Input: part model. Units: mm. Frame: model coordinates. A direction names the side the tool comes from. Give positions to 0.01 mm unless a question says otherwise; leave off trailing zeros. Loops run counter-clockwise (first coordinate to the right, second up) from the corner with the lowest first, then second, coordinate; pieces in that order, holes last. Notation, with made-up numbers: (-19.75, -36) -> (27.25, -36) arc R20 ccw to (27.25, -23) -> close; hole circle Ø8 at (51.25, 77.25). An arc over 180 degrees is marked (long way). One line per question, with ' | ' between items.
from build123d import *

# Parameters (mm, degrees)
F0_W          = 55.7
F0_H          = 13.4
F1_DEPTH      = 1.6
F2_W          = 55.7
F2_H          = 13.4
F2_W_2        = 26
F2_H_2        = 6
F3_DEPTH      = 4
F4_W          = 8
F4_H          = 10
F5_DEPTH      = 3
F6_T1_DEPTH   = 70.7
F7_W          = 6
F7_H          = 3.5
F8_DEPTH      = 10
F9_R          = 2
F10_T4_DEPTH  = 21.4300979278
F10_T10_DEPTH = 41.4300979278
F10_T16_DEPTH = 41.4300979278
F10_T22_DEPTH = 21.4300979278
F11_C1_SIZE   = 2
F11_C2_SIZE   = 2


# Not quite as in the source:
# - a fillet or chamfer that OpenCascade refuses, or shapes differently, is made with other operations: its cross-section is extruded or revolved along the edge and cut away or added


with BuildPart() as f1:
    # F0 (on Top) → F1 (new body)
    with BuildSketch(Plane.XY):
        with Locations((-20.85, 5.5)):
            Rectangle(F0_W, F0_H)
        Polygon((1, 0), (0, 0), (-47.5, 0), (-47.5, 11), (0, 11), (1, 11), align=None, mode=Mode.SUBTRACT)
    extrude(amount=F1_DEPTH)

    # F2 (on face) → F3 (join)
    with BuildSketch(Plane.XY.offset(1.6)):
        with Locations((-20.85, 5.5)):
            Rectangle(F2_W, F2_H)
        Polygon((-47.5, 0.5), (-47.5, 10.5), (-47.5, 11), (1, 11), (1, 0), (-47.5, 0), align=None, mode=Mode.SUBTRACT)
        Polygon((-47.5, 11), (-47.5, 10.5), (-31.5, 10.5), (-31.5, 0.5), (-47.5, 0.5), (-47.5, 0), (1, 0), (1, 11), align=None)
        with Locations((-13, 5.5)):
            Rectangle(F2_W_2, F2_H_2, mode=Mode.SUBTRACT)
    extrude(amount=F3_DEPTH)

    # F4 (on face) → F5 (join)
    with BuildSketch(Plane.XY.offset(5.6)):
        Polygon((-39.5, 12.2), (-48.7, 12.2), (-48.7, -1.2), (-39.5, -1.2), (-39.5, 0.5), (-47.5, 0.5), (-47.5, 10.5), (-39.5, 10.5), align=None)
        with Locations((-43.5, 5.5)):
            Rectangle(F4_W, F4_H)
    extrude(amount=-F5_DEPTH)

    # F6: fillet of radius 3 on 2 edges, made by hand

    # F6_s2 → F6_t1 (cut)
    with BuildSketch(Plane.YZ.offset(-56.2)):
        with BuildLine():
            ThreePointArc((12.2, 2.6), (11.3213203436, 4.7213203436), (9.2, 5.6))
            Line((9.2, 5.6), (12.2, 5.6))
            Line((12.2, 5.6), (12.2, 2.6))
        make_face()
        with BuildLine():
            ThreePointArc((1.8, 5.6), (-0.3213203436, 4.7213203436), (-1.2, 2.6))
            Line((-1.2, 2.6), (-1.2, 5.6))
            Line((-1.2, 5.6), (1.8, 5.6))
        make_face()
    extrude(amount=F6_T1_DEPTH, mode=Mode.SUBTRACT)

    # F7 (on face) → F8 (cut)
    with BuildSketch(Plane(origin=(-48.7, 0, 0), x_dir=(0, -1, 0), z_dir=(-1, 0, 0))):
        with Locations((-5.5, 1.75)):
            Rectangle(F7_W, F7_H)
    extrude(amount=-F8_DEPTH, mode=Mode.SUBTRACT)

    # F9
    f9_edges = [f1.edges().sort_by_distance(p)[0] for p in [
        (-44.1, 8.5, 3.5),
        (-44.1, 2.5, 3.5),
    ]]
    fillet(f9_edges, radius=F9_R)

    # F10: chamfer of 3 on 4 edges, made by hand


with BuildPart() as f10_tool2:
    # F10_s3 → F10_t4 (new body)
    with BuildSketch(Plane.XZ.offset(5.2150489639)):
        Polygon((-29, 5.6), (-26, 2.6), (-26, 5.6), align=None)
    extrude(amount=-F10_T4_DEPTH)

    split(bisect_by=Plane(origin=(0, 2.55, 2.55), x_dir=(1, 0, 0), z_dir=(0, 0.7071067812, 0.7071067812)), keep=Keep.TOP)

    split(bisect_by=Plane(origin=(0, 2.95, -2.95), x_dir=(1, 0, 0), z_dir=(0, -0.7071067812, 0.7071067812)), keep=Keep.TOP)


with BuildPart() as f1_1:
    add(f1.part)

    # F10_t1: cut F10_tool2
    add(f10_tool2.part, mode=Mode.SUBTRACT)


with BuildPart() as f10_tool8:
    # F10_s9 → F10_t10 (new body)
    with BuildSketch(Plane.YZ.offset(-33.7150489639)):
        Polygon((11.5, 5.6), (8.5, 2.6), (8.5, 5.6), align=None)
    extrude(amount=F10_T10_DEPTH)

    split(bisect_by=Plane(origin=(-11.7, 0, -11.7), x_dir=(0, 1, 0), z_dir=(0.7071067812, 0, 0.7071067812)), keep=Keep.TOP)

    split(bisect_by=Plane(origin=(-1.3, 0, 1.3), x_dir=(0, 1, 0), z_dir=(-0.7071067812, 0, 0.7071067812)), keep=Keep.TOP)


with BuildPart() as f1_2:
    add(f1_1.part)

    # F10_t7: cut F10_tool8
    add(f10_tool8.part, mode=Mode.SUBTRACT)


with BuildPart() as f10_tool14:
    # F10_s15 → F10_t16 (new body)
    with BuildSketch(Plane.YZ.offset(7.7150489639)):
        Polygon((-0.5, 5.6), (2.5, 2.6), (2.5, 5.6), align=None)
    extrude(amount=-F10_T16_DEPTH)

    split(bisect_by=Plane(origin=(-11.7, 0, -11.7), x_dir=(0, 1, 0), z_dir=(0.7071067812, 0, 0.7071067812)), keep=Keep.TOP)

    split(bisect_by=Plane(origin=(-1.3, 0, 1.3), x_dir=(0, 1, 0), z_dir=(-0.7071067812, 0, 0.7071067812)), keep=Keep.TOP)


with BuildPart() as f1_3:
    add(f1_2.part)

    # F10_t13: cut F10_tool14
    add(f10_tool14.part, mode=Mode.SUBTRACT)


with BuildPart() as f10_tool20:
    # F10_s21 → F10_t22 (new body)
    with BuildSketch(Plane.XZ.offset(-16.2150489639)):
        Polygon((3, 5.6), (0, 2.6), (0, 5.6), align=None)
    extrude(amount=F10_T22_DEPTH)

    split(bisect_by=Plane(origin=(0, 2.55, 2.55), x_dir=(1, 0, 0), z_dir=(0, 0.7071067812, 0.7071067812)), keep=Keep.TOP)

    split(bisect_by=Plane(origin=(0, 2.95, -2.95), x_dir=(1, 0, 0), z_dir=(0, -0.7071067812, 0.7071067812)), keep=Keep.TOP)


with BuildPart() as f1_4:
    add(f1_3.part)

    # F10_t19: cut F10_tool20
    add(f10_tool20.part, mode=Mode.SUBTRACT)

    # F11: chamfer of 2 on 3 edges, made by hand

    # F11_c1
    f11_c1_edges = [f1_4.edges().sort_by_distance(p)[0] for p in [
        (-31.5, 5.5, 1.6),
    ]]
    chamfer(f11_c1_edges, length=F11_C1_SIZE)

    # F11_c2
    f11_c2_edges = [f1_4.edges().sort_by_distance(p)[0] for p in [
        (-39.5, 9.3351646544, 2.6),
    ]]
    chamfer(f11_c2_edges, length=F11_C2_SIZE)


solid = f1_4.part
1. Section query C-C (x = -35). Output: boundary loops of the cut face in (y, z).
Determined:
outline: (-1.2, 0) -> (0, 0) -> (0, 1.6) -> (0.5, 1.6) -> (0.5, 5.3) arc R3 ccw to (-1.2, 2.6) -> close; (10.5, 1.6) -> (11, 1.6) -> (11, 0) -> (12.2, 0) -> (12.2, 2.6) arc R3 ccw to (10.5, 5.3) -> close
2. Section query D-D (z = 0.85). Output: boundary loops of the cut face in (x, y), then the cut area to 3 significant figures.
Determined:
outline: (-48.7, -1.2) -> (7, -1.2) -> (7, 12.2) -> (-48.7, 12.2) -> (-48.7, 8.5) -> (-47.5, 8.5) -> (-47.5, 11) -> (1, 11) -> (1, 0) -> (-47.5, 0) -> (-47.5, 2.5) -> (-48.7, 2.5) -> close | area: 206 mm2
3. Pin query (flat end, axial travel): P1, Ø0.5, axis at y = 5.5, z = 2, coming from the -X side; P2, Ø1.9, axis at x = -46, y = 9.5, coming from the -Z side; P3, Ø1.9, axis at x = -39.5, z = 3.5, coming from the +Y side; P4, Ø0.8, axis at y = 8, z = 0.5, coming from the -X side. Return the tip coordinate at first contact, or that it passes through.
Determined:
P1: stops at x = -30.15 | P2: stops at z = 2.6 | P3: stops at y = 12.2 | P4: stops at x = 1
4. Reachability of faces 1 (the flat face through (-18, 2, 1.6)), 2 (the cylindrical face through (-44.6, 3.3, 3.1)), 3 (the flat face through (0, 5, 2)) from +Z, -Z, +X, -X, +Y, -Y: full face, straight path, thin tool, end or side. Return the list, or none.
Determined:
face 1: -Z | face 2: -Z, -X | face 3: +Z, -Z
5. Pull-direction query (Y, two-part tool) for faces 4 (the flat face through (-48, 2.5, 1)), 5 (the flat face through (-30, 6, 5.6)), 6 (the cylindrical face through (-21.24, -0.638, 4.348)); classes: pulls with the +Y half, pulls with the -Y half, needs draft (parallel to the pull), parting line crosses it, or undercut.
Determined:
face 4: undercut | face 5: needs draft | face 6: pulls with the -Y half
6. Section query A-A (x = -5.5). Output: boundary loops of the cut face in (y, z), then the cut area to 3 significant figures.
Determined:
outline: (-1.2, 0) -> (0, 0) -> (0, 1.6) -> (2.5, 1.6) -> (2.5, 2.6) -> (0.06, 5.04) arc R3 ccw to (-1.2, 2.6) -> close; (8.5, 1.6) -> (11, 1.6) -> (11, 0) -> (12.2, 0) -> (12.2, 2.6) arc R3 ccw to (10.94, 5.04) -> (8.5, 2.6) -> close | area: 21.5 mm2
7. Section query B-B (y = 6). Output: boundary loops of the cut face in (x, z), then the cut area to 3 significant figures.
Determined:
outline: (-48.7, 3.5) -> (-40.6, 3.5) -> (-39.5, 4.6) -> (-39.5, 5.6) -> (-48.7, 5.6) -> close; (-31.5, 3.6) -> (-29.5, 1.6) -> (-26, 1.6) -> (-26, 2.6) -> (-29, 5.6) -> (-31.5, 5.6) -> close; (0, 1.6) -> (1, 1.6) -> (1, 0) -> (7, 0) -> (7, 5.6) -> (3, 5.6) -> (0, 2.6) -> close | area: 67.3 mm2
8. Ray query, line 1 along Y through (x, z) = (-22, 1.4); line 2 along X through (y, z) = (10, 0.25); line 3 along X through (y, z) = (2.5, 2.75). Return the intervals inside material, ascending. Write a range as from..to.
Determined:
line 1: y = -1.2..0, 11..12.2 | line 2: x = -48.7..-47.5, 1..7 | line 3: x = -48.7..-41.35, -30.65..-26.15, 0.15..7
